```python
from build123d import *

# Parameters (mm, degrees)
SKETCH_1_R      = 2.75
SKETCH_1_R_2    = 2
EXTRUDE_1_DEPTH = 5
EXTRUDE_START   = -1
SKETCH_2_R      = 3
SKETCH_2_R_2    = 2
EXTRUDE_2_DEPTH = 1
SKETCH_3_R      = 3.012416382
SKETCH_3_R_2    = 2
EXTRUDE_3_DEPTH = 1


with BuildPart() as part:
    # 草图1 → 凸台-拉伸1 (new body)
    with BuildSketch(Plane.XY):
        Circle(SKETCH_1_R)
        Circle(SKETCH_1_R_2, mode=Mode.SUBTRACT)
    extrude(amount=EXTRUDE_1_DEPTH)

    # 草图2 → 凸台-拉伸2 (add)
    with BuildSketch(Plane.XY.offset(5).offset(EXTRUDE_START)):
        Circle(SKETCH_2_R)
        Circle(SKETCH_2_R_2, mode=Mode.SUBTRACT)
    extrude(amount=EXTRUDE_2_DEPTH)

    # 草图3 → 凸台-拉伸3 (add)
    with BuildSketch(Plane(origin=(0, 0, 0), x_dir=(-1, 0, 0), z_dir=(0, 0, -1))):
        Circle(SKETCH_3_R)
        with Locations(Location((0, 0, 0), (0, 0, 180))):
            Circle(SKETCH_3_R_2, mode=Mode.SUBTRACT)
    extrude(amount=-EXTRUDE_3_DEPTH)


solid = part.part
```
Here's how the part is built. I have some questions about the finished solid (model axes, mm). A direction names the side the tool comes from. Give positions to 0.01 mm unless a question says otherwise; leave off trailing zeros. Loops run counter-clockwise (first coordinate to the right, second up) from the corner with the lowest first, then second, coordinate; pieces in that order, holes last. Notation, with made-up numbers: M -3.5,55.25 L 35.5,55.25 A19 ccw 35.5,60.25 Z; hole C -20,26.5 d7. An arc over 180 degrees is marked long. Use one line per item in the form item = value. Start each with the question number.
Q1. If we section it at D-D (y = 2.5): Write out the boundary of the cut face in (x, z), then the cut area to 3 significant figures.
Q2. Thinking about a two-plate mould opening in Z: for faces 1 (the cylindrical face through (-0.596, -2.685, 2.479)), 2 (the flat face through (-2, -1, 0)), 3 (the flat face through (1, -2, 5)), 4 (the cylindrical face through (3.01, 0.13, 0.49)), which applies, +Z half, -Z half, draft (parallel to the pull), parting line (faces both ways), or undercut?
Q3. Will these pins go through, and if not, where does the flat tip stop? pin 1 Ø2 at (x, y) = (-2.5, -1.5) entering from -Z; pin 2 Ø3.5 at (x, y) = (0, 0) entering from -Z.
Q4. If we section it at C-C (z = 0.45): Write out the boundary of the cut face in (x, y), then the cut area to 3 significant figures.
Q5. I need wall thicknesses on line 1 along Y through (x, z) = (0, 1.25); line 2 along X through (y, z) = (0.75, 2.9); line 3 along X through (y, z) = (1.5, 0.55). Which ranges of each line are inside material? Lowest first, please.
Q6. If we section it at A-A (x = 0): Write out the boundary of the cut face in (y, z), then the cut area to 3 significant figures.
Q7. Which directions (+Z, -Z, +X, -X, +Y, -Y) give clear straight access to the entire face, cutting with the end or side of a thin tool? Please do faces 5 (the cylindrical face through (-3, 0.1, 4.5)), 6 (the cylindrical face through (0, -2, 2)).
Taken from the geometry:
q1.outline = M -1.68,0 L 1.68,0 L 1.68,1 L 1.15,1 L 1.15,4 L 1.66,4 L 1.66,5 L -1.66,5 L -1.66,4 L -1.15,4 L -1.15,1 L -1.68,1 Z
q1.area = 13.6 mm^2
q2.face_1 = undercut
q2.face_2 = -Z half
q2.face_3 = +Z half
q2.face_4 = draft
q3.pin_1 = 0
q3.pin_2 = through
q4.outline = C 0,0 d6.02; hole C 0,0 d4
q4.area = 15.9 mm^2
q5.line_1 = -2.75 to -2, 2 to 2.75
q5.line_2 = -2.65 to -1.85, 1.85 to 2.65
q5.line_3 = -2.61 to -1.32, 1.32 to 2.61
q6.outline = M -3.01,0 L -2,0 L -2,5 L -3,5 L -3,4 L -2.75,4 L -2.75,1 L -3.01,1 Z; M 2,0 L 3.01,0 L 3.01,1 L 2.75,1 L 2.75,4 L 3,4 L 3,5 L 2,5 Z
q6.area = 8.52 mm^2
q7.face_5 = +Z
q7.face_6 = +Z, -Z
